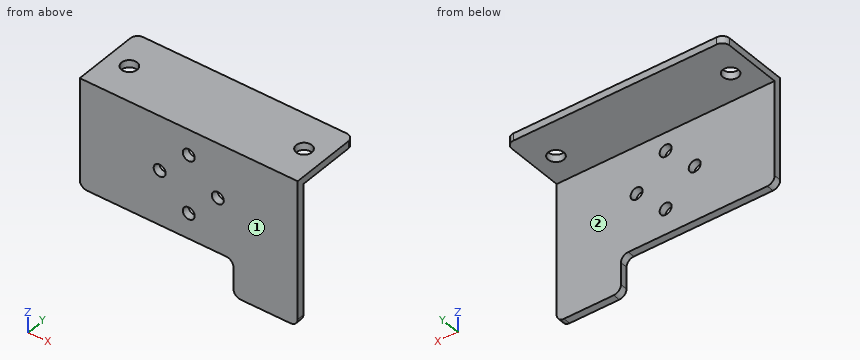
```python
from build123d import *

# Parameters (mm, degrees)
SKETCH_1_W      = 60
SKETCH_1_H      = 30
SKETCH_1_R      = 1.65
EXTRUDE_3_DEPTH = 2
SKETCH_3_W      = 60
SKETCH_3_H      = 20
SKETCH_3_R      = 2.15
EXTRUDE_4_DEPTH = 2
SKETCH_4_W      = 17.695256038
SKETCH_4_H      = 10
EXTRUDE_5_DEPTH = 2
FILLET_1_R      = 2
FILLET_2_R      = 2
FILLET_3_R      = 2
FILLET_4_R      = 2
FILLET_5_R      = 2
FILLET_6_R      = 2


with BuildPart() as part:
    # 草图1 → 凸台-拉伸3 (new body)
    with BuildSketch(Plane(origin=(0, 0, 0), x_dir=(1, 0, 0), z_dir=(0, 1, 0))):
        Rectangle(SKETCH_1_W, SKETCH_1_H)
        with Locations((0, 8)):
            Circle(SKETCH_1_R, mode=Mode.SUBTRACT)
        with Locations((0, -8)):
            Circle(SKETCH_1_R, mode=Mode.SUBTRACT)
        with Locations((8, 0)):
            Circle(SKETCH_1_R, mode=Mode.SUBTRACT)
        with Locations((-8, 0)):
            Circle(SKETCH_1_R, mode=Mode.SUBTRACT)
    extrude(amount=EXTRUDE_3_DEPTH)

    # 草图3 → 凸台-拉伸4 (add)
    with BuildSketch(Plane.XY.offset(15)):
        with Locations((0, 10)):
            Rectangle(SKETCH_3_W, SKETCH_3_H)
        with Locations((24, 10)):
            Circle(SKETCH_3_R, mode=Mode.SUBTRACT)
        with Locations((-24.08, 10)):
            Circle(SKETCH_3_R, mode=Mode.SUBTRACT)
    extrude(amount=-EXTRUDE_4_DEPTH)

    # 草图4 → 凸台-拉伸5 (add)
    with BuildSketch(Plane(origin=(0, 2, 0), x_dir=(1, 0, 0), z_dir=(0, 1, 0))):
        with Locations((21.152371981, 20)):
            Rectangle(SKETCH_4_W, SKETCH_4_H)
    extrude(amount=-EXTRUDE_5_DEPTH)

    # 圆角1
    fillet_1_edges = [part.edges().sort_by_distance(p)[0] for p in [
        (30, 1, -25),
    ]]
    fillet(fillet_1_edges, radius=FILLET_1_R)

    # 圆角2
    fillet_2_edges = [part.edges().sort_by_distance(p)[0] for p in [
        (12.304743962, 1, -25),
    ]]
    fillet(fillet_2_edges, radius=FILLET_2_R)

    # 圆角3
    fillet_3_edges = [part.edges().sort_by_distance(p)[0] for p in [
        (12.304743962, 1, -15),
    ]]
    fillet(fillet_3_edges, radius=FILLET_3_R)

    # 圆角4
    fillet_4_edges = [part.edges().sort_by_distance(p)[0] for p in [
        (-30, 1, -15),
    ]]
    fillet(fillet_4_edges, radius=FILLET_4_R)

    # 圆角5
    fillet_5_edges = [part.edges().sort_by_distance(p)[0] for p in [
        (-30, 20, 14),
    ]]
    fillet(fillet_5_edges, radius=FILLET_5_R)

    # 圆角6
    fillet_6_edges = [part.edges().sort_by_distance(p)[0] for p in [
        (30, 20, 14),
    ]]
    fillet(fillet_6_edges, radius=FILLET_6_R)


solid = part.part
```
Check sheet for the modelled part. Datum: model origin and axes. Units: mm. Face numbers are marked on the shaded views. A direction names the side the tool comes from. Coordinates: 2 decimals unless noted, no trailing zeros. Loops run counter-clockwise (first coordinate to the right, second up) from the corner with the lowest first, then second, coordinate; pieces in that order, holes last. Notation, with made-up numbers: M 34,31 L 65,31 A16 cw 65,38 Z; hole C 72.25,85 d8. An arc over 180 degrees is marked long. Answer as a JSON object with one key per item and string values.
1. Access from +Z, -Z, +X, -X, +Y, -Y to the whole of each face (thin tool, end or side, straight path). Record for the marked faces 1 and 2.
Outcome:
{"face 1": "+Z, -Z, +X, -X, -Y", "face 2": "-Z, +X, -X, +Y"}
2. Sectioned sample at B-B on x = 24. Record the cut outline in (y, z), and give its area (3 significant figures).
Outcome:
{"outline": "M 0,-25 L 2,-25 L 2,13 L 7.85,13 L 7.85,15 L 0,15 Z; M 12.15,13 L 20,13 L 20,15 L 12.15,15 Z", "area": "107 mm²"}
3. Scan lines: L1, parallel to Z at x = 8, y = 1.3; L2, parallel to X at y = 0.55, z = 0; L3, parallel to Y at x = 24, z = 14. Record each from-to range of solid material in increasing order. Write a range as from..to.
Outcome:
{"L1": "-15..-1.65, 1.65..15", "L2": "-30..-9.65, -6.35..6.35, 9.65..30", "L3": "0..7.85, 12.15..20"}
4. Depth check by flat-ended pin: P1, Ø1.5, axis at x = 2.5, y = 10, coming from the -Z side; P2, Ø0.6, axis at x = -17, y = 1.5, coming from the -Z side; P3, Ø10, axis at x = -13.5, z = -11.5, coming from the +Y side. Enter the tip coordinate at first touch or a pass-through.
Outcome:
{"P1": "z = 13", "P2": "z = -15", "P3": "y = 2"}
5. Sectioned sample at A-A on z = 8. Record the cut outline in (x, y), and give its area (3 significant figures).
Outcome:
{"outline": "M -30,0 L -1.65,0 L -1.65,2 L -30,2 Z; M 1.65,0 L 30,0 L 30,2 L 1.65,2 Z", "area": "113 mm²"}
6. Sectioned sample at C-C on y = 11.5. Record the cut outline in (x, z), and give its area (3 significant figures).
Outcome:
{"outline": "M -30,13 L -25.62,13 L -25.62,15 L -30,15 Z; M -22.54,13 L 22.46,13 L 22.46,15 L -22.54,15 Z; M 25.54,13 L 30,13 L 30,15 L 25.54,15 Z", "area": "108 mm²"}
7. Sectioned sample at D-D on x = 17.5. Record the cut outline in (y, z).
Outcome:
{"outline": "M 0,-25 L 2,-25 L 2,13 L 20,13 L 20,15 L 0,15 Z"}
